Input: dimensioned drawing with shaded views. Units: mm. Origin: part minimum x, y, z. A direction names the side the tool comes from. Give positions to 0.01 mm unless a question says otherwise; leave off trailing zeros. Order: outer loops, then holes, each group sorted by start corner. A loop starts at its lowest first (then second) coordinate and runs counter-clockwise, first axis right, second up.
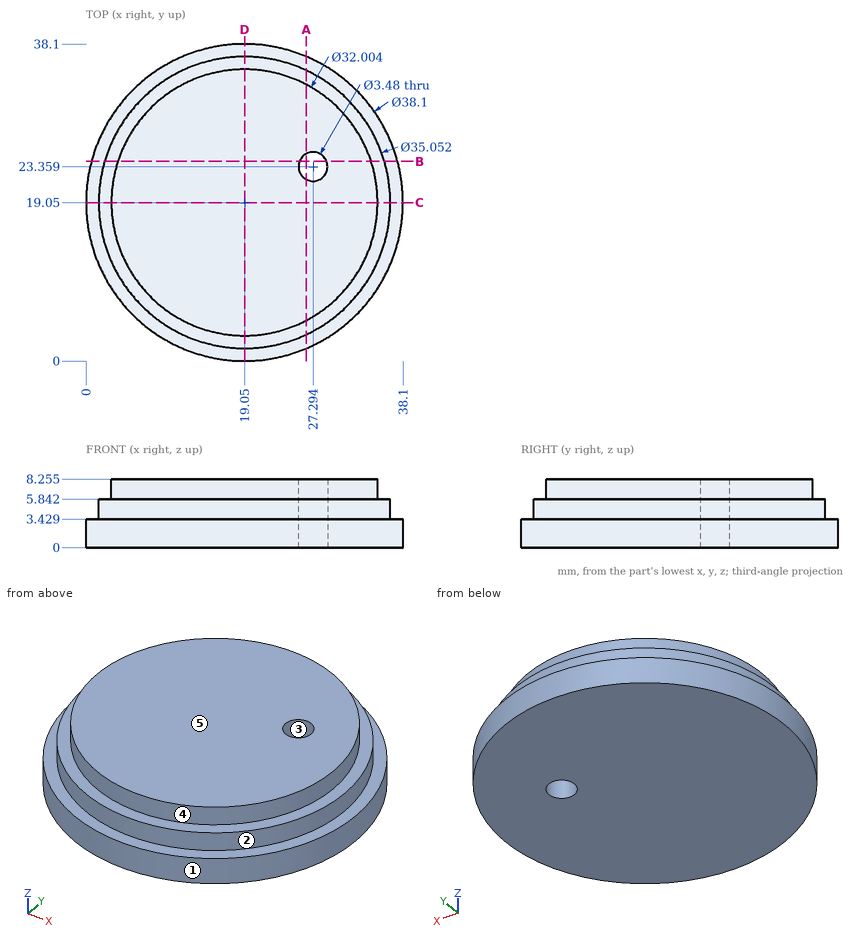
1) Draft query along Y for the marked faces 3, 4 and 5. Return one class per face: +Y half, -Y half, draft (parallel to the pull), parting line (faces both ways), or undercut.
Report:
face 3: undercut
face 4: parting line
face 5: draft
2) Pin query (flat end, axial travel): pin 1 (1.5 mm diameter, centred on y = 22.5, z = 1.5, fed in from -X); pin 2 (3 mm diameter, centred on x = 27.29, y = 23.36, fed in from +Z); pin 3 (2 mm diameter, centred on x = 4.5, z = 7, fed in from +Y); pin 4 (3 mm diameter, centred on x = 17, z = 5, fed in from +Y). Return the tip coordinate at first contact, or that it passes through.
Report:
pin 1: stops at x = 0.19
pin 2: passes through
pin 3: stops at y = 27.56
pin 4: stops at y = 36.57
3) Section query C-C, the plane y = 19.05. Return the cut outline in (x, z) (1 decimal).
Report:
outline: (0, 0) - (38.1, 0) - (38.1, 3.4) - (36.6, 3.4) - (36.6, 5.8) - (35.1, 5.8) - (35.1, 8.3) - (3, 8.3) - (3, 5.8) - (1.5, 5.8) - (1.5, 3.4) - (0, 3.4) - close
4) Reachability of the marked faces 1 and 2 from +Z, -Z, +X, -X, +Y, -Y: full face, straight path, thin tool, end or side. Return the list, or none.
Report:
face 1: +Z, -Z
face 2: +Z
5) Section query B-B, the plane y = 24. Return the cut outline in (x, z) (1 decimal), and give its area (3 significant figures).
Report:
outline: (0.7, 0) - (25.7, 0) - (25.7, 8.3) - (3.8, 8.3) - (3.8, 5.8) - (2.2, 5.8) - (2.2, 3.4) - (0.7, 3.4) - close; (28.9, 0) - (37.4, 0) - (37.4, 3.4) - (35.9, 3.4) - (35.9, 5.8) - (34.3, 5.8) - (34.3, 8.3) - (28.9, 8.3) - close
area: 254 mm2
6) Material intervals for L1, parallel to Z at x = 12, y = 35; L2, parallel to Y at x = 27.5, z = 4.25 (1 decimal); L3, parallel to Y at x = 19.5, z = 6 (1 decimal), sorted ascending.
Report:
L1: z = 0 to 5.84
L2: y = 3.7 to 21.6, 25.1 to 34.4
L3: y = 3.1 to 35
7) Section query A-A, the plane x = 26.5. Return the cut outline in (y, z) (1 decimal).
Report:
outline: (1.5, 0) - (21.8, 0) - (21.8, 8.3) - (4.9, 8.3) - (4.9, 5.8) - (3.2, 5.8) - (3.2, 3.4) - (1.5, 3.4) - close; (24.9, 0) - (36.6, 0) - (36.6, 3.4) - (34.9, 3.4) - (34.9, 5.8) - (33.2, 5.8) - (33.2, 8.3) - (24.9, 8.3) - close
